from build123d import *

# Parameters (mm, degrees)
F1_DEPTH       = 76.2
F3_DEPTH       = 25.4
F4_R           = 32.5001429767
F8_D           = 25.4
F8_CBORE_D     = 38.1
F8_CBORE_DEPTH = 6.35
F10_DEPTH      = 25.4
F12_DEPTH      = 25.4
F14_DEPTH      = 6.35


# Not quite as in the source:
# - a feature names something its author has since deleted; it is built from what else it names


with BuildPart() as f1:
    # F0 (on Front) → F1 (new body, symmetric)
    with BuildSketch(Plane.XZ):
        Polygon((5.1541254637, -56.7420329794), (5.1541254637, 95.6579670206), (-24.9778814614, 96.1331352592), (-24.9778814614, -31.3420329794), (-71.0458745363, -31.3420329794), (-71.0458745363, -56.7420329794), align=None)
    extrude(amount=F1_DEPTH, both=True)

    # F2 (on face) → F3 (cut)
    with BuildSketch(Plane.XY.offset(-31.3420329794)):
        with BuildLine():
            Line((-71.0458745363, 12.1218512269), (-71.0458745363, -13.2781487731))
            Line((-71.0458745363, -13.2781487731), (-58.3458745363, -13.2781487731))
            ThreePointArc((-58.3458745363, -13.2781487731), (-45.6458745363, -0.5781487731), (-58.3458745363, 12.1218512269))
            Line((-58.3458745363, 12.1218512269), (-71.0458745363, 12.1218512269))
        make_face()
    extrude(amount=-F3_DEPTH, mode=Mode.SUBTRACT)

    # F4
    f4_edges = [f1.edges().sort_by_distance(p)[0] for p in [
        (-9.911878, 76.2, 95.895551),
        (-9.911878, -76.2, 95.895551),
    ]]
    fillet(f4_edges, radius=F4_R)

    # F8 (through all)
    with Locations(Plane(origin=(-24.9778814614, 0, 0), x_dir=(0, -1, 0), z_dir=(-1, 0, 0))):
        with Locations((0, 44.6130335331)):
            CounterBoreHole(F8_D / 2, F8_CBORE_D / 2, F8_CBORE_DEPTH)

    # F9 (on face) → F10 (join)
    with BuildSketch(Plane.XZ.offset(38.1)):
        Polygon((-24.9547883868, -31.3420329794), (-24.9778814614, 63.6289514861), (-45.6458745363, -31.3420329794), align=None)
    extrude(amount=F10_DEPTH)

    # F11 (on face) → F12 (join)
    with BuildSketch(Plane(origin=(0, 38.1, 0), x_dir=(-1, 0, 0), z_dir=(0, 1, 0))):
        Polygon((45.6458745363, -31.3420329794), (24.9778814614, 63.6289514861), (24.9778814614, -31.3420329794), align=None)
    extrude(amount=F12_DEPTH)

    # F13 (on face) → F14 (join)
    with BuildSketch(Plane.XY.offset(-31.3420329794)):
        with BuildLine():
            Line((-71.0458745363, 18.4718512269), (-71.0458745363, 12.1218512269))
            Line((-71.0458745363, 12.1218512269), (-58.3458745363, 12.1218512269))
            ThreePointArc((-58.3458745363, 12.1218512269), (-45.6458745363, -0.5781487731), (-58.3458745363, -13.2781487731))
            Line((-58.3458745363, -13.2781487731), (-71.0458745363, -13.2781487731))
            Line((-71.0458745363, -13.2781487731), (-71.0458745363, -19.6281487731))
            Line((-71.0458745363, -19.6281487731), (-58.3458745363, -19.6281487731))
            ThreePointArc((-58.3458745363, -19.6281487731), (-39.2958745363, -0.5781487731), (-58.3458745363, 18.4718512269))
            Line((-58.3458745363, 18.4718512269), (-71.0458745363, 18.4718512269))
        make_face()
    extrude(amount=F14_DEPTH)


solid = f1.part
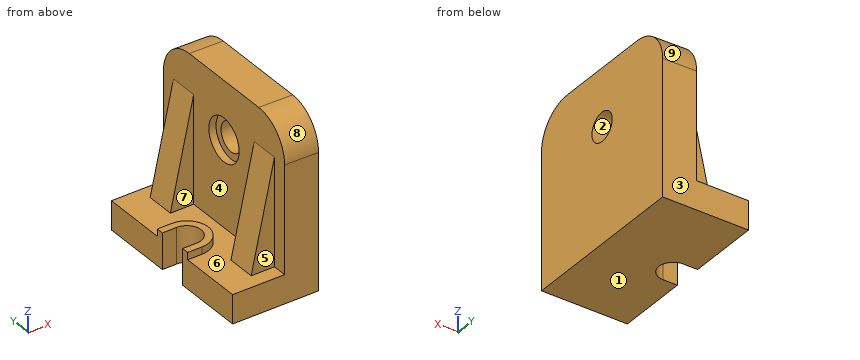
Geometry: final body of the model. Coordinates: model frame, mm. Face numbers are marked on the shaded views. A direction names the side the tool comes from. Coordinates: 2 decimals unless noted, no trailing zeros. Loops run counter-clockwise (first coordinate to the right, second up) from the corner with the lowest first, then second, coordinate; pieces in that order, holes last. Notation, with made-up numbers: (22, 65) - (53, 65) arc R3 cw to (53, 70) - close; hole circle Ø5 at (30.25, 46). An arc over 180 degrees is marked (long way). One line per question, with ' | ' between items. Start each with the question number.
(1) Cut plane C-C on y = 9.5. Output: boundary loops of the cut face in (x, z), and give its area (3 significant figures).
(2) Ray query, L1, parallel to X at y = -13.5, z = 30; L2, parallel to Z at x = -53, y = 25; L3, parallel to Y at x = -32, z = 7. Return the intervals inside material, ascending. Write a range as from..to.
(3) Cut plane A-A on z = 51.5. Output: boundary loops of the cut face in (x, y).
(4) Cut plane B-B on x = -52.5. Output: boundary loops of the cut face in (y, z), and give its area (3 significant figures).
(5) First-contact query: pin 1 (2 mm diameter, centred on x = -45, z = -18, fed in from +Y); pin 2 (1.9 mm diameter, centred on x = -63.5, z = -28.5, fed in from -Y); pin 3 (6 mm diameter, centred on x = -34, z = -3.5, fed in from +Y); pin 4 (16 mm diameter, centred on x = -56.5, y = -6.5, fed in from +Z). Flat tips, straight axial feed; report the tip coordinate or a pass-through.
(6) Cut plane D-D on z = -43.5. Output: boundary loops of the cut face in (x, y), and give its area (3 significant figures).
(7) Draft query along Y for the marked faces 1, 2, 3 and 4. Return one class per face: +Y half, -Y half, draft (parallel to the pull), parting line (faces both ways), or undercut.
(8) Reachability of the marked faces 5, 6, 7, 8 and 9 from +Z, -Z, +X, -X, +Y, -Y: full face, straight path, thin tool, end or side. Return the list, or none.
Here are the results:
1) outline: (-50.62, -56.74) - (5.15, -56.74) - (5.15, 36.18) - (-18.63, 36.18) - (-18.63, 28.1) - (-24.98, 28.1) - (-24.98, -31.34) - (-42.18, -31.34) - (-42.18, -24.99) - (-50.62, -24.99) - close; (-24.98, 61.13) - (-18.63, 61.13) - (-18.63, 53.04) - (5.15, 53.04) - (5.15, 95.66) - (-24.98, 96.13) - close | area: 4,690 mm²
2) L1: -24.98..5.15 | L2: -56.74..-31.34 | L3: -63.5..-38.1, 38.1..63.5
3) outline: (-27.62, -63.5) - (-24.98, -63.5) - (-24.98, -76.2) - (5.15, -76.2) - (5.15, -10.67) - (-18.63, -10.67) - (-18.63, -17.76) - (-24.98, -17.76) - (-24.98, -38.1) - (-27.62, -38.1) - close; (-27.62, 38.1) - (-24.98, 38.1) - (-24.98, 17.76) - (-18.63, 17.76) - (-18.63, 10.67) - (5.15, 10.67) - (5.15, 76.2) - (-24.98, 76.2) - (-24.98, 63.5) - (-27.62, 63.5) - close
4) outline: (-76.2, -56.74) - (-11.85, -56.74) - (-11.85, -24.99) - (-18.71, -24.99) - (-18.71, -31.34) - (-76.2, -31.34) - close; (10.7, -56.74) - (76.2, -56.74) - (76.2, -31.34) - (17.55, -31.34) - (17.55, -24.99) - (10.7, -24.99) - close | area: 3,390 mm²
5) pin 1: through | pin 2: y = -19.63 | pin 3: y = 63.5 | pin 4: z = -24.99
6) outline: (-71.05, -76.2) - (5.15, -76.2) - (5.15, 76.2) - (-71.05, 76.2) - (-71.05, 12.12) - (-58.35, 12.12) arc R12.7 cw to (-58.35, -13.28) - (-71.05, -13.28) - close | area: 11,000 mm²
7) face 1: draft | face 2: undercut | face 3: +Y half | face 4: undercut
8) face 5: +Z, -X, -Y | face 6: +Z | face 7: +Z, -X | face 8: +Z, +X, -Y | face 9: +Z, +X, +Y
